Input: part model. Units: mm. Frame: model coordinates. Round coordinates to 2 decimals unless told otherwise and drop trailing zeros. Order: outer loops, then holes, each group sorted by start corner. A loop starts at its lowest first (then second) coordinate and runs counter-clockwise, first axis right, second up. Notation, with made-up numbers: (29, 14) -> (50, 14) arc R22 cw to (50, 36) -> close; hole circle Ø10 at (67.25, -1). An arc over 180 degrees is marked (long way). Use a Markdown table: item, result.
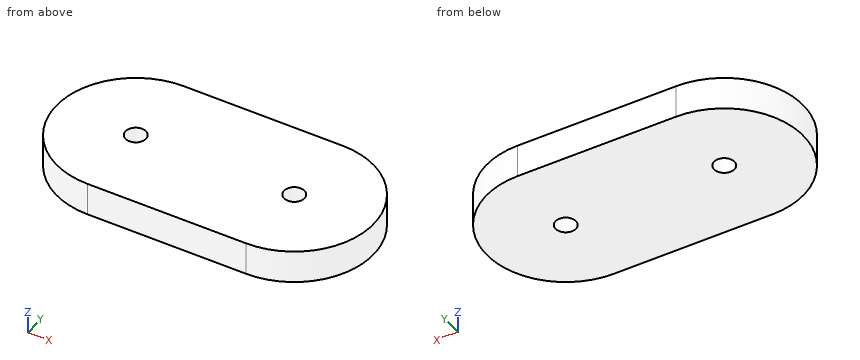
from build123d import *

# Parameters (mm, degrees)
EXTRUDE_1_DEPTH     = 5
SKETCH_2_R          = 1.55
CUT_EXTRUDE_1_DEPTH = 12


with BuildPart() as part:
    # 草图1 → 凸台-拉伸1 (new body)
    with BuildSketch(Plane.XY):
        with BuildLine():
            Line((0, 12), (24, 12))
            ThreePointArc((24, 12), (36, 0), (24, -12))
            Line((24, -12), (0, -12))
            ThreePointArc((0, -12), (-12, 0), (0, 12))
        make_face()
    extrude(amount=EXTRUDE_1_DEPTH)

    # 草图2 → 切除-拉伸1 (cut)
    with BuildSketch(Plane(origin=(0, 0, 0), x_dir=(-1, 0, 0), z_dir=(0, 0, -1))):
        Circle(SKETCH_2_R)
        with Locations((-24, 0)):
            Circle(SKETCH_2_R)
    extrude(amount=-CUT_EXTRUDE_1_DEPTH, mode=Mode.SUBTRACT)


solid = part.part
1) Cut plane B-B on z = 2.85. Return loops of the section in (x, y), and give its area (3 significant figures).
Results found:
| item | result |
|---|---|
| outline | (0, -12) -> (24, -12) arc R12 ccw to (24, 12) -> (0, 12) arc R12 ccw to start; hole circle Ø3.1 at (0, 0); hole circle Ø3.1 at (24, 0) |
| area | 1,010 mm² |
2) Cut plane A-A on y = 0. Return loops of the section in (x, z), and give its area (3 significant figures).
Results found:
| item | result |
|---|---|
| outline | (-12, 0) -> (-1.55, 0) -> (-1.55, 5) -> (-12, 5) -> close; (1.55, 0) -> (22.45, 0) -> (22.45, 5) -> (1.55, 5) -> close; (25.55, 0) -> (36, 0) -> (36, 5) -> (25.55, 5) -> close |
| area | 209 mm² |
3) Pin query (flat end, axial travel): pin 1 Ø3 at (y, z) = (4, 4) entering from +X; pin 2 Ø1.9 at (x, y) = (0, 0) entering from -Z. Return the tip coordinate at first contact, or that it passes through.
Results found:
| item | result |
|---|---|
| pin 1 | stops at x = 35.74 |
| pin 2 | passes through |
4) Line query: L1, parallel to Y at x = 24, z = 1.75; L2, parallel to X at y = 0.75, z = 0.9; L3, parallel to Y at x = 23, z = 1.45. Output: solid intervals per line, ascending. Write a range as [from, to].
Results found:
| item | result |
|---|---|
| L1 | y = [-12, -1.55], [1.55, 12] |
| L2 | x = [-11.98, -1.36], [1.36, 22.64], [25.36, 35.98] |
| L3 | y = [-12, -1.18], [1.18, 12] |
5) Cut plane C-C on x = 23.5. Return loops of the section in (y, z), and give its area (3 significant figures).
Results found:
| item | result |
|---|---|
| outline | (-12, 0) -> (-1.47, 0) -> (-1.47, 5) -> (-12, 5) -> close; (1.47, 0) -> (12, 0) -> (12, 5) -> (1.47, 5) -> close |
| area | 105 mm² |
6) Cut plane D-D on x = 1. Return loops of the section in (y, z).
Results found:
| item | result |
|---|---|
| outline | (-12, 0) -> (-1.18, 0) -> (-1.18, 5) -> (-12, 5) -> close; (1.18, 0) -> (12, 0) -> (12, 5) -> (1.18, 5) -> close |
